Read the model definition and answer for the solid it produces. Units are mm, in the model's axes. A direction names the side the tool comes from. Coordinates: 2 decimals unless noted, no trailing zeros. Order: outer loops, then holes, each group sorted by start corner. A loop starts at its lowest first (then second) coordinate and runs counter-clockwise, first axis right, second up. Notation, with made-up numbers: M -2,-14 L 23,-14 A22 cw 23,15 Z; hole C 36,-6.75 d10. An arc over 180 degrees is marked long. Write each question's results on one line, items separated by ' | '.
```python
from build123d import *

# Parameters (mm, degrees)
SKETCH1_W           = 58.166
SKETCH1_H           = 73.66
BOSS_EXTRUDE1_DEPTH = 5.08
SKETCH2_W           = 27.686
SKETCH2_H           = 5.08
CUT_EXTRUDE1_DEPTH  = 94.994071919
SKETCH7_R           = 6
CUT_EXTRUDE2_DEPTH  = 94.994071919
FILLET1_R           = 21.59
FILLET2_R           = 12.7


with BuildPart() as part:
    # Sketch1 → Boss-Extrude1 (new body)
    with BuildSketch(Plane.XY):
        with Locations((29.083, 36.83)):
            Rectangle(SKETCH1_W, SKETCH1_H)
    extrude(amount=BOSS_EXTRUDE1_DEPTH)

    # Sketch2 → Cut-Extrude1 (cut, through all)
    with BuildSketch(Plane.XY.offset(5.08)):
        with Locations((29.083, 66.04)):
            Rectangle(SKETCH2_W, SKETCH2_H)
    extrude(amount=-CUT_EXTRUDE1_DEPTH, mode=Mode.SUBTRACT)

    # Sketch7 → Cut-Extrude2 (cut, through all)
    with BuildSketch(Plane.XY.offset(5.08)):
        with Locations((29.083, 35.9)):
            Circle(SKETCH7_R)
    extrude(amount=-CUT_EXTRUDE2_DEPTH, mode=Mode.SUBTRACT)

    # Fillet1
    fillet1_edges = [part.edges().sort_by_distance(p)[0] for p in [
        (58.166, 0, 2.54),
        (0, 0, 2.54),
    ]]
    fillet(fillet1_edges, radius=FILLET1_R)

    # Fillet2
    fillet2_edges = [part.edges().sort_by_distance(p)[0] for p in [
        (0, 73.66, 2.54),
        (58.166, 73.66, 2.54),
    ]]
    fillet(fillet2_edges, radius=FILLET2_R)


solid = part.part
```
(1) The part is cut by section A-A, the plane y = 35.9. Write down the section's boundary in (x, z), then the cut area to 3 significant figures.
Conclusion:
outline: M 0,0 L 23.08,0 L 23.08,5.08 L 0,5.08 Z; M 35.08,0 L 58.17,0 L 58.17,5.08 L 35.08,5.08 Z | area: 235 mm²
(2) The part is cut by section D-D, the plane y = 11. Write down the section's boundary in (x, z).
Conclusion:
outline: M 2.78,0 L 55.39,0 L 55.39,5.08 L 2.78,5.08 Z
(3) Straight lines are drawn through the part: line 1 (Y direction, x = 34, z = 3.55); line 2 (Y direction, x = 38.5, z = 2.55); line 3 (Y direction, x = 43.5, z = 3.95). For each, find the intervals that lie inside material, in ascending order.
Conclusion:
line 1: 0 to 32.46, 39.34 to 63.5, 68.58 to 73.66 | line 2: 0.09 to 63.5, 68.58 to 73.66 | line 3: 1.14 to 73.66
(4) For faces 4 (the cylindrical face through (54.347, 70.038, 2.576)), 5 (the flat face through (29, 68.58, 3)), determine the directions among +Z, -Z, +X, -X, +Y, -Y from which every point of the face is accessible in a straight line to the end or side of a thin tool.
Conclusion:
face 4: +Z, -Z, +X, +Y | face 5: +Z, -Z
(5) The part is cut by section B-B, the plane z = 3.1. Write down the section's boundary in (x, y), then the cut area to 3 significant figures.
Conclusion:
outline: M 0,21.59 A21.59 ccw 21.59,0 L 36.58,0 A21.59 ccw 58.17,21.59 L 58.17,60.96 A12.7 ccw 45.47,73.66 L 12.7,73.66 A12.7 ccw 0,60.96 Z; hole M 15.24,63.5 L 42.93,63.5 L 42.93,68.58 L 15.24,68.58 Z; hole C 29.08,35.9 d12 | area: 3,760 mm²
(6) Given pin 1 (1 mm diameter, centred on x = 16.5, z = 4.5, fed in from -Y); pin 2 (1.5 mm diameter, centred on y = 67, z = 2.5, fed in from +X); pin 3 (1 mm diameter, centred on x = 7, z = 4.5, fed in from -Y); pin 4 (12 mm diameter, centred on x = 13, y = 22, fed in from -Z), each flat-ended and moving along its own axis, determine where each tip first touches the part or whether it passes through.
Conclusion:
pin 1: y = 0.49 | pin 2: x = 57.01 | pin 3: y = 5.23 | pin 4: z = 0
(7) The mould has two halves that part along Y. Classify faces 1 (the flat face through (42.926, 66, 3)), 2 (the cylindrical face through (51.674, 6.157, 2.576)), 3 (the flat face through (35.1, 37.3, 5.08)): pulls with the +Y half, pulls with the -Y half, needs draft (parallel to the pull), parting line crosses it, or undercut.
Conclusion:
face 1: undercut | face 2: pulls with the -Y half | face 3: needs draft
(8) The part is cut by section C-C, the plane x = 20. Write down the section's boundary in (y, z), then the cut area to 3 significant figures.
Conclusion:
outline: M 0.06,0 L 63.5,0 L 63.5,5.08 L 0.06,5.08 Z; M 68.58,0 L 73.66,0 L 73.66,5.08 L 68.58,5.08 Z | area: 348 mm²
